The listing builds one solid part. Answer for the finished solid, in the listing's coordinates (mm). A direction names the side the tool comes from. Round coordinates to 2 decimals unless told otherwise and drop trailing zeros. Order: outer loops, then holes, each group sorted by start corner. A loop starts at its lowest first (then second) coordinate and runs counter-clockwise, first axis right, second up. Notation, with made-up numbers: (29, -37.5) -> (64, -37.5) arc R20 ccw to (64, -21.5) -> close; hole circle Ø9 at (-3.5, -18.5). An arc over 180 degrees is marked (long way). Return JSON: item names as keys, results as strings. Group by question number.
(1) Consider line 1 (Z direction, x = -9, y = 10.75) (3 decimals); line 2 (Y direction, x = 11, z = -252.5) (3 decimals); line 3 (X direction, y = -11.25, z = -316.23). Determine where each line is inside the solid, lowest interval first. Write a range as [from, to].
(2) Each of these flat-tipped pins is pushed along its axis until it touches: pin 1 (3 mm diameter, centred on x = 12.7, z = -238.125, fed in from -Y); pin 2 (3 mm diameter, centred on x = -11.81, z = 308.86, fed in from +Y) (3 decimals); pin 3 (4.5 mm diameter, centred on x = 12.62, z = -299.72, fed in from -Y) (3 decimals). Where does it stop, or does it pass through?
(3) Which of the six approach directions +Z, -Z, +X, -X, +Y, -Y give full straight-line access (tool end or side, diameter ignored) to faces 5 (the face through (0, -9.525, -5)), 6 (the face through (0.568, 9.711, -159.366)), 7 (the face through (0.349, -11.09, -169.855))?
(4) Determine the mould class of faces 1 (the face through (0.57, 9.71, 110.51)), 2 (the face through (0, -12.7, -4)), 3 (the face through (0, 10, -320.675)), 4 (the face through (-4.83, -11.09, 101.65)) for opening direction Z: +Z half, -Z half, draft (parallel to the pull), parting line (faces both ways), or undercut.
(5) The part is cut by section B-B (y = 5). Determine the outline of the cut face in (x, z) (3 decimals), plus the area to 3 significant figures.
(6) The part is cut by section A-A (z = -197). Determine the outline of the cut face in (x, y) (3 decimals), plus the area to 3 significant figures.
from build123d import *

# Parameters (mm, degrees)
BOSS_EXTRUDE1_DEPTH              = 320.675
BOSS_EXTRUDE1_DEPTH_BACK         = 320.675
SKETCH3_W                        = 50.8
SKETCH3_H                        = 25.4
SKETCH3_W_2                      = 44.45
SKETCH3_H_2                      = 19.05
CUT_EXTRUDE1_DEPTH               = 323.680609311
CUT_EXTRUDE1_DEPTH_BACK          = 323.680609311
F_10_CLEARANCE_HOLE1_D           = 4.9784
F_10_CLEARANCE_HOLE1_DEPTH       = 5.08
F_10_CLEARANCE_HOLE1_TIP         = 1.495662253
F_10_CLEARANCE_HOLE3_D           = 4.9784
F_10_CLEARANCE_HOLE3_DEPTH       = 5.08
F_10_CLEARANCE_HOLE3_TIP         = 1.495662253
F_10_CLEARANCE_HOLE4_D           = 4.9784
F_1_4_CLEARANCE_HOLE1_D          = 6.5278
F_1_4_CLEARANCE_HOLE1_DEPTH      = 5.08
F_1_4_CLEARANCE_HOLE1_TIP        = 1.961148974
F_10_CLEARANCE_HOLE5_D           = 4.9784
F_10_CLEARANCE_HOLE5_DEPTH       = 5.08
F_10_CLEARANCE_HOLE5_CSINK_D     = 10.4394
F_10_CLEARANCE_HOLE5_CSINK_ANGLE = 82
F_10_CLEARANCE_HOLE5_TIP         = 1.495662253
SKETCH25_R                       = 7.9375
CUT_EXTRUDE2_DEPTH               = 323.44622226


with BuildPart() as part:
    # Sketch3 → Boss-Extrude1 (new, two sides: drawn at the far end of the back side and taken through both)
    with BuildSketch(Plane.XY.offset(-BOSS_EXTRUDE1_DEPTH_BACK)):
        Rectangle(SKETCH3_W, SKETCH3_H)
        Rectangle(SKETCH3_W_2, SKETCH3_H_2, mode=Mode.SUBTRACT)
    extrude(amount=BOSS_EXTRUDE1_DEPTH + BOSS_EXTRUDE1_DEPTH_BACK)

    # Sketch4 → Cut-Extrude1 (cut, two sides: drawn at the far end of the back side and taken through both)
    with BuildSketch(Plane(origin=(0, 12.7, 0), x_dir=(1, 0, 0), z_dir=(0, 1, 0)).offset(-CUT_EXTRUDE1_DEPTH_BACK)):
        Polygon((1322.117470931, -320.675), (25.4, -320.675), (-25.4, -320.675), (25.4, -305.627354456), (1268.718301677, 62.660305034), (3837.350959621, 420.474595165), (3890.750128875, 37.139290131), align=None)
    extrude(amount=CUT_EXTRUDE1_DEPTH + CUT_EXTRUDE1_DEPTH_BACK, mode=Mode.SUBTRACT)

    # #10 Clearance Hole1
    with Locations(Plane(origin=(0, 12.7, 0), x_dir=(1, 0, 0), z_dir=(0, 1, 0))):
        with Locations((-11.811, -275.746327933), (-11.811, -308.859955913), (11.811, -297.574221755), (12.047235668, -264.390617583)):
            Hole(F_10_CLEARANCE_HOLE1_D / 2, depth=F_10_CLEARANCE_HOLE1_DEPTH)
            with Locations((0, 0, -(F_10_CLEARANCE_HOLE1_DEPTH + F_10_CLEARANCE_HOLE1_TIP / 2))):  # 118° drill point
                Cone(0, F_10_CLEARANCE_HOLE1_D / 2, F_10_CLEARANCE_HOLE1_TIP, mode=Mode.SUBTRACT)

    # #10 Clearance Hole3
    with Locations(Plane(origin=(0, -12.7, 0), x_dir=(-1, 0, 0), z_dir=(0, -1, 0))):
        with Locations((-12.6238, 299.72), (12.7762, 299.72), (12.7762, 316.23), (-12.6238, 316.23)):
            Hole(F_10_CLEARANCE_HOLE3_D / 2, depth=F_10_CLEARANCE_HOLE3_DEPTH)
            with Locations((0, 0, -(F_10_CLEARANCE_HOLE3_DEPTH + F_10_CLEARANCE_HOLE3_TIP / 2))):  # 118° drill point
                Cone(0, F_10_CLEARANCE_HOLE3_D / 2, F_10_CLEARANCE_HOLE3_TIP, mode=Mode.SUBTRACT)

    # #10 Clearance Hole4 (through all)
    with Locations(Plane(origin=(0, -12.7, 0), x_dir=(-1, 0, 0), z_dir=(0, -1, 0))):
        with Locations((-12.7, 238.125), (12.7, 238.125), (12.7, 212.725), (-12.7, 212.725), (-14.622625311, 277.25194622), (-14.622625311, 258.20194622)):
            Hole(F_10_CLEARANCE_HOLE4_D / 2)

    # 1/4 Clearance Hole1
    with Locations(Plane(origin=(0, 12.7, 0), x_dir=(1, 0, 0), z_dir=(0, 1, 0))):
        with Locations((-10.8204, 173.0375), (10.8204, 173.0375), (10.8204, 150.8125), (-10.8204, 150.8125), (-10.8204, -96.8375), (10.8204, -96.8375), (-10.8204, -119.0625), (10.8204, -119.0625)):
            Hole(F_1_4_CLEARANCE_HOLE1_D / 2, depth=F_1_4_CLEARANCE_HOLE1_DEPTH)
            with Locations((0, 0, -(F_1_4_CLEARANCE_HOLE1_DEPTH + F_1_4_CLEARANCE_HOLE1_TIP / 2))):  # 118° drill point
                Cone(0, F_1_4_CLEARANCE_HOLE1_D / 2, F_1_4_CLEARANCE_HOLE1_TIP, mode=Mode.SUBTRACT)

    # #10 Clearance Hole5
    with Locations(Plane(origin=(0, 12.7, 0), x_dir=(1, 0, 0), z_dir=(0, 1, 0))):
        with Locations((0, -107.95), (0, 161.925)):
            CounterSinkHole(F_10_CLEARANCE_HOLE5_D / 2, F_10_CLEARANCE_HOLE5_CSINK_D / 2, depth=F_10_CLEARANCE_HOLE5_DEPTH, counter_sink_angle=F_10_CLEARANCE_HOLE5_CSINK_ANGLE)
            with Locations((0, 0, -(F_10_CLEARANCE_HOLE5_DEPTH + F_10_CLEARANCE_HOLE5_TIP / 2))):  # 118° drill point
                Cone(0, F_10_CLEARANCE_HOLE5_D / 2, F_10_CLEARANCE_HOLE5_TIP, mode=Mode.SUBTRACT)

    # Sketch25 → Cut-Extrude2 (cut, through all)
    with BuildSketch(Plane(origin=(0, -9.525, 0), x_dir=(1, 0, 0), z_dir=(0, 1, 0))):
        with Locations(Location((0, -107.95, 0), (0, 0, 270))):
            Circle(SKETCH25_R)
        with Locations(Location((0, 161.925, 0), (0, 0, 270))):
            Circle(SKETCH25_R)
    extrude(amount=-CUT_EXTRUDE2_DEPTH, mode=Mode.SUBTRACT)


solid = part.part
Answer below:
{
 "1": {"line 1": "z = [-320.675, -175.747], [-170.328, -153.522], [-148.103, 94.128], [99.547, 116.353], [121.772, 315.817]", "line 2": "y = [-12.7, -9.525], [9.525, 12.7]", "line 3": "x = [-25.4, -15.27], [-10.29, 10.13], [15.11, 25.4]"},
 "2": {"pin 1": "passes through", "pin 2": "stops at y = -9.525", "pin 3": "stops at y = 9.525"},
 "3": {"face 5": "+Z, -Z", "face 6": "+Y", "face 7": "-Y"},
 "4": {"face 1": "undercut", "face 2": "draft", "face 3": "-Z half", "face 4": "undercut"},
 "5": {"outline": "(-25.4, -320.675) -> (-22.225, -320.675) -> (-22.225, 319.735) -> (-25.4, 320.675) -> close; (22.225, -320.675) -> (25.4, -320.675) -> (25.4, 305.627) -> (22.225, 306.568) -> close", "area": "4,020 mm²"},
 "6": {"outline": "(-25.4, -12.7) -> (25.4, -12.7) -> (25.4, 12.7) -> (-25.4, 12.7) -> close; hole (-22.225, -9.525) -> (22.225, -9.525) -> (22.225, 9.525) -> (-22.225, 9.525) -> close", "area": "444 mm²"}
}
